```python
from build123d import *

# Parameters (mm, degrees)
AUFSATZ_LINEAR_AUSTRAGEN1_DEPTH                      = 150
STIRNSENKUNG_F_R_M2_FLACHKOPFSCHRAUBE_MI_D           = 2.4
STIRNSENKUNG_F_R_M2_FLACHKOPFSCHRAUBE_MI_CBORE_D     = 5
STIRNSENKUNG_F_R_M2_FLACHKOPFSCHRAUBE_MI_CBORE_DEPTH = 1.6


with BuildPart() as part:
    # Skizze1 → Aufsatz-Linear austragen1 (new body)
    with BuildSketch(Plane.XY):
        Polygon((0, 0), (-6.5, 0), (-6.5, 3.3), (-2.5, 3.3), (-2.5, 6.3), (-6, 7.3), (-6, 8.6), (-2, 8.6), (-2, 8.1), (2, 8.1), (2, 8.6), (6, 8.6), (6, 7.3), (2.5, 6.3), (2.5, 3.3), (6.5, 3.3), (6.5, 0), align=None)
    extrude(amount=AUFSATZ_LINEAR_AUSTRAGEN1_DEPTH)

    # Stirnsenkung für M2 Flachkopfschraube mit Schlitz1 (through all)
    with Locations(Plane(origin=(0, 0, 0), x_dir=(-1, 0, 0), z_dir=(0, -1, 0))):
        with Locations((0, -85), (0, -60), (0, -35), (0, -10), (0, -110), (0, -135)):
            CounterBoreHole(STIRNSENKUNG_F_R_M2_FLACHKOPFSCHRAUBE_MI_D / 2, STIRNSENKUNG_F_R_M2_FLACHKOPFSCHRAUBE_MI_CBORE_D / 2, STIRNSENKUNG_F_R_M2_FLACHKOPFSCHRAUBE_MI_CBORE_DEPTH)


solid = part.part
```
CAD build for the part. Positions are in the model's coordinates, mm. A direction names the side the tool comes from. Round coordinates to 2 decimals unless told otherwise and drop trailing zeros. Loops run counter-clockwise (first coordinate to the right, second up) from the corner with the lowest first, then second, coordinate; pieces in that order, holes last. Notation, with made-up numbers: M -21.5,83 L 15.5,83 A19 ccw 15.5,87 Z; hole C -20,57.25 d1. An arc over 180 degrees is marked long. Return JSON: item names as keys, results as strings. Group by question number.
(1) Mould opens along X. For faces 6 (the cylindrical face through (-0.26, 4.9, 136.17)), 7 (the flat face through (0, 0, 74)), 8 (the flat face through (6.5, 2, 74)), 9 (the flat face through (-1, 1.6, 84)) say: +X half, -X half, draft (parallel to the pull), parting line (faces both ways), or undercut.
(2) Tool access for faces 1 (the flat face through (0, 3, 150)), 2 (the cylindrical face through (0.54, 0.79, 12.44)), 3 (the flat face through (4.274, 6.807, 73.95)), 4 (the flat face through (-5, 3.3, 74)), 5 (the flat face through (0, 8.1, 74)): list every direction of +Z, -Z, +X, -X, +Y, -Y with a clear straight run to the whole face (end or side of a thin tool).
(3) Drop flat-ended pins along their axis: P1, Ø1.5, axis at x = -1, z = 35, coming from the -Y side; P2, Ø3, axis at x = -4, z = 79, coming from the -Y side; P3, Ø1, axis at y = 8, z = 61, coming from the +X side; P4, Ø3, axis at x = 0, z = 85, coming from the +Y side. Give the stop position or say it passes through.
(4) Wall check: probe 1 along X at (y, z) = (0.7, 110); probe 2 along X at (y, z) = (3.5, 22.5); probe 3 along Y at (x, z) = (-3.75, 75). Give the ranges that are in metal, low to high. Write a range as [from, to].
(5) Saw through at C-C, the plane x = 4.5. List the corners of the cut face in (y, z).
(6) Saw through at B-B, the plane z = 99.5. List the corners of the cut face in (x, y), and give its area (3 significant figures).
(7) Saw through at A-A, the plane y = 5. List the corners of the cut face in (x, z), and give its area (3 significant figures).
Answer list:
{
 "1": {"face 6": "undercut", "face 7": "draft", "face 8": "+X half", "face 9": "undercut"},
 "2": {"face 1": "+Z, +X, -X, +Y, -Y", "face 2": "-Y", "face 3": "+Z, -Z, +X", "face 4": "+Z, -Z, -X", "face 5": "+Z, -Z, +Y"},
 "3": {"P1": "y = 1.6", "P2": "y = 0", "P3": "x = 6", "P4": "y = 8.1"},
 "4": {"probe 1": "[-6.5, -2.5], [2.5, 6.5]", "probe 2": "[-2.5, 2.5]", "probe 3": "[0, 3.3], [6.66, 8.6]"},
 "5": {"outline": "M 0,0 L 3.3,0 L 3.3,150 L 0,150 Z; M 6.87,0 L 8.6,0 L 8.6,150 L 6.87,150 Z"},
 "6": {"outline": "M -6.5,0 L 6.5,0 L 6.5,3.3 L 2.5,3.3 L 2.5,6.3 L 6,7.3 L 6,8.6 L 2,8.6 L 2,8.1 L -2,8.1 L -2,8.6 L -6,8.6 L -6,7.3 L -2.5,6.3 L -2.5,3.3 L -6.5,3.3 Z", "area": "80.0 mm2"},
 "7": {"outline": "M -2.5,0 L 2.5,0 L 2.5,150 L -2.5,150 Z; hole C 0,10 d2.4; hole C 0,35 d2.4; hole C 0,60 d2.4; hole C 0,85 d2.4; hole C 0,110 d2.4; hole C 0,135 d2.4", "area": "723 mm2"}
}
